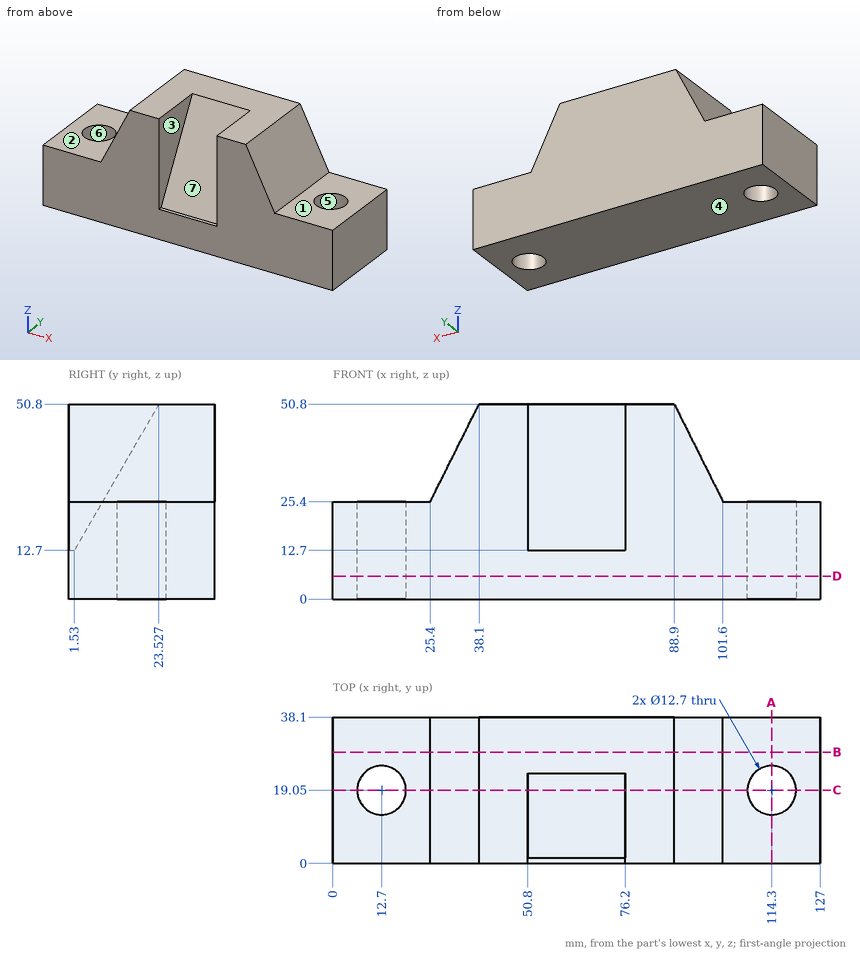
Check sheet for the drawn part. Datum: minimum x, y, z corner. Units: mm. A direction names the side the tool comes from. Coordinates: 2 decimals unless noted, no trailing zeros. Write each loop counter-clockwise with the first axis right and the second up, starting at its lowest first coordinate (ties: lowest second). Pieces come first, ordered by that corner, then holes. Notation, with made-up numbers: (31.25, 2) - (51.25, 2) arc R33 ccw to (51.25, 36) - close; hole circle Ø1 at (69, 42.5). An arc over 180 degrees is marked (long way). Answer as a JSON object with one key per item and string values.
(1) Thickness scan on line 1 along X through (y, z) = (19, 16); line 2 along X through (y, z) = (24.5, 24.5); line 3 along Y through (x, z) = (114.3, 14). Record the ranges inside material, lowest first.
Report:
{"line 1": "0 to 6.35, 19.05 to 107.95, 120.65 to 127", "line 2": "0 to 9.44, 15.96 to 111.04, 117.56 to 127", "line 3": "0 to 12.7, 25.4 to 38.1"}
(2) Gauge pin test, flat ends, axial feed: pin 1 Ø7.5 at (x, y) = (114.3, 19.05) entering from +Z; pin 2 Ø5 at (y, z) = (29, 35) entering from +X; pin 3 Ø1 at (y, z) = (4, 39.5) entering from -X; pin 4 Ø12 at (x, y) = (28.5, 5) entering from +Z. Record the tip position at first contact, or that the pin passes through.
Report:
{"pin 1": "through", "pin 2": "x = 98.05", "pin 3": "x = 32.2", "pin 4": "z = 43.6"}
(3) Cross-section at A-A on x = 114.3. Record the cut outline in (y, z), plus the area to 3 significant figures.
Report:
{"outline": "(0, 0) - (12.7, 0) - (12.7, 25.4) - (0, 25.4) - close; (25.4, 0) - (38.1, 0) - (38.1, 25.4) - (25.4, 25.4) - close", "area": "645 mm^2"}
(4) Tool access check on the marked faces 1, 2 and 3. Record the directions out of +Z, -Z, +X, -X, +Y, -Y that give a thin tool (end or side, any length) a straight path to the whole face; none if there is none.
Report:
{"face 1": "+Z, +X, +Y, -Y", "face 2": "+Z, -X, +Y, -Y", "face 3": "+Z, -Y"}
(5) Cross-section at C-C on y = 19.05. Record the cut outline in (x, z).
Report:
{"outline": "(0, 0) - (6.35, 0) - (6.35, 25.4) - (0, 25.4) - close; (19.05, 0) - (107.95, 0) - (107.95, 25.4) - (101.6, 25.4) - (88.9, 50.8) - (76.2, 50.8) - (76.2, 43.05) - (50.8, 43.05) - (50.8, 50.8) - (38.1, 50.8) - (25.4, 25.4) - (19.05, 25.4) - close; (120.65, 0) - (127, 0) - (127, 25.4) - (120.65, 25.4) - close"}
(6) Mould release check, pull along Y, two halves, no side actions. Record for the marked faces 4, 5, 6 and 7: pulls with the +Y half, pulls with the -Y half, needs draft (parallel to the pull), parting line crosses it, or undercut.
Report:
{"face 4": "needs draft", "face 5": "undercut", "face 6": "undercut", "face 7": "pulls with the -Y half"}
(7) Cross-section at B-B on y = 29. Record the cut outline in (x, z), plus the area to 3 significant figures.
Report:
{"outline": "(0, 0) - (127, 0) - (127, 25.4) - (101.6, 25.4) - (88.9, 50.8) - (38.1, 50.8) - (25.4, 25.4) - (0, 25.4) - close", "area": "4,840 mm^2"}
(8) Cross-section at D-D on z = 6. Record the cut outline in (x, y), plus the area to 3 significant figures.
Report:
{"outline": "(0, 0) - (127, 0) - (127, 38.1) - (0, 38.1) - close; hole circle Ø12.7 at (12.7, 19.05); hole circle Ø12.7 at (114.3, 19.05)", "area": "4,590 mm^2"}
